```python
from build123d import *

# Parameters (mm, degrees)
CROQUIS1_R              = 5
SALIENTE_EXTRUIR1_DEPTH = 170
CORTAR_EXTRUIR1_START   = -5.5
CROQUIS2_R              = 5
CROQUIS2_R_2            = 4.75
CORTAR_EXTRUIR1_DEPTH   = 5.5
CROQUIS3_R              = 5
CROQUIS3_R_2            = 4.75
CORTAR_EXTRUIR2_DEPTH   = 5.5
CHAFL_N1_SIZE           = 0.5
CORTAR_EXTRUIR4_DEPTH   = 3.5


with BuildPart() as part:
    # Croquis1 → Saliente-Extruir1 (new body)
    with BuildSketch(Plane.XY):
        Circle(CROQUIS1_R)
    extrude(amount=SALIENTE_EXTRUIR1_DEPTH)

    # Croquis2 → Cortar-Extruir1 (cut)
    with BuildSketch(Plane.XY.offset(170).offset(CORTAR_EXTRUIR1_START)):
        Circle(CROQUIS2_R)
        Circle(CROQUIS2_R_2, mode=Mode.SUBTRACT)
    extrude(amount=CORTAR_EXTRUIR1_DEPTH, mode=Mode.SUBTRACT)

    # Croquis3 → Cortar-Extruir2 (cut)
    with BuildSketch(Plane(origin=(0, 0, 0), x_dir=(-1, 0, 0), z_dir=(0, 0, -1))):
        Circle(CROQUIS3_R)
        with Locations(Location((0, 0, 0), (0, 0, 180))):
            Circle(CROQUIS3_R_2, mode=Mode.SUBTRACT)
    extrude(amount=-CORTAR_EXTRUIR2_DEPTH, mode=Mode.SUBTRACT)

    # Chaflán1
    chafl_n1_edges = [part.edges().sort_by_distance(p)[0] for p in [
        (-4.75, 0, 0),
        (-4.75, 0, 170),
    ]]
    chamfer(chafl_n1_edges, length=CHAFL_N1_SIZE)

    # Croquis4 → Cortar-Extruir4 (cut)
    with BuildSketch(Plane(origin=(0, 5, 0), x_dir=(-1, 0, 0), z_dir=(0, -1, 0))):
        with BuildLine():
            Line((2, -117.5), (2, -152.5))
            ThreePointArc((2, -152.5), (0, -154.5), (-2, -152.5))
            Line((-2, -152.5), (-2, -117.5))
            ThreePointArc((-2, -117.5), (0, -115.5), (2, -117.5))
        make_face()
        with BuildLine():
            Line((-2, -102.5), (-2, -67.5))
            ThreePointArc((-2, -67.5), (0, -65.5), (2, -67.5))
            Line((2, -67.5), (2, -102.5))
            ThreePointArc((2, -102.5), (0, -104.5), (-2, -102.5))
        make_face()
    extrude(amount=CORTAR_EXTRUIR4_DEPTH, mode=Mode.SUBTRACT)


solid = part.part
```
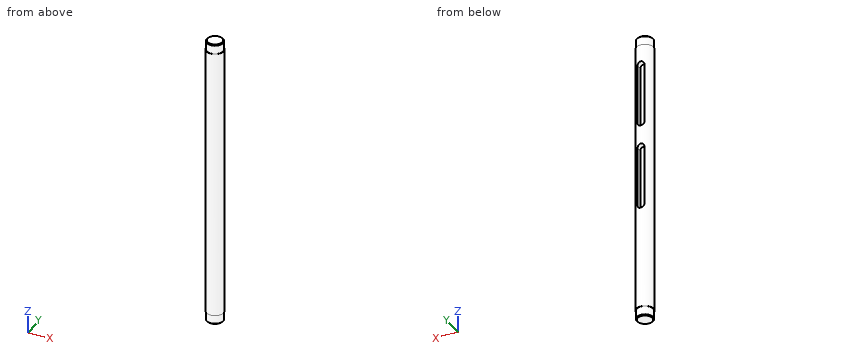
The listing builds one solid part. Answer for the finished solid, in the listing's coordinates (mm). Give positions to 0.01 mm unless a question says otherwise; leave off trailing zeros. Loops run counter-clockwise (first coordinate to the right, second up) from the corner with the lowest first, then second, coordinate; pieces in that order, holes last. Notation, with made-up numbers: (39.5, 18.25) - (52.5, 18.25) arc R23 cw to (52.5, 56.25) - close; hole circle Ø8 at (6.5, 0.25). An arc over 180 degrees is marked (long way). Answer as CSV lines item,"result". Start each with the question number.
Item 1: A cutting plane is placed at B-B on z = 96. Determine the outline of the cut face in (x, y), then the cut area to 3 significant figures.
Item 2: A cutting plane is placed at A-A on x = 0. Determine the outline of the cut face in (y, z).
Item 3: Each of these flat-tipped pins is pushed along its axis until it touches: pin 1 (3 mm diameter, centred on x = -1.5, y = 2, fed in from -Z); pin 2 (1.5 mm diameter, centred on y = 3.5, z = 135, fed in from +X); pin 3 (0.9 mm diameter, centred on y = 3, z = 142, fed in from -X); pin 4 (4 mm diameter, centred on y = -4, z = 117.5, fed in from -X). Where does it stop, or does it pass through?
Item 4: Find the intervals of material crossed by line 1 (Z direction, x = -0.5, y = 2); line 2 (Z direction, x = 1.25, y = 1.75); line 3 (X direction, y = 2, z = 130.5), in increasing order. Write a range as from..to.
Item 5: A cutting plane is placed at C-C on z = 52.5. Determine the outline of the cut face in (x, y), then the cut area to 3 significant figures.
Found:
1,outline,"(-2, 1.5) - (-2, 4.58) arc R5 ccw (long way) to (2, 4.58) - (2, 1.5) - close"
1,area,"65.1 mm^2"
2,outline,"(-5, 5.5) - (-4.75, 5.5) - (-4.75, 0.5) - (-4.25, 0) - (4.25, 0) - (4.75, 0.5) - (4.75, 5.5) - (5, 5.5) - (5, 65.5) - (1.5, 65.5) - (1.5, 104.5) - (5, 104.5) - (5, 115.5) - (1.5, 115.5) - (1.5, 154.5) - (5, 154.5) - (5, 164.5) - (4.75, 164.5) - (4.75, 169.5) - (4.25, 170) - (-4.25, 170) - (-4.75, 169.5) - (-4.75, 164.5) - (-5, 164.5) - close"
3,pin 1,"stops at z = 0"
3,pin 2,"stops at x = 4.18"
3,pin 3,"stops at x = -4.3"
3,pin 4,"stops at x = -4.58"
4,line 1,"z = 0..65.56, 104.44..115.56, 154.44..170"
4,line 2,"z = 0..65.94, 104.06..115.94, 154.06..170"
4,line 3,"x = -4.58..-2, 2..4.58"
5,outline,"circle Ø10 at (0, 0)"
5,area,"78.5 mm^2"
